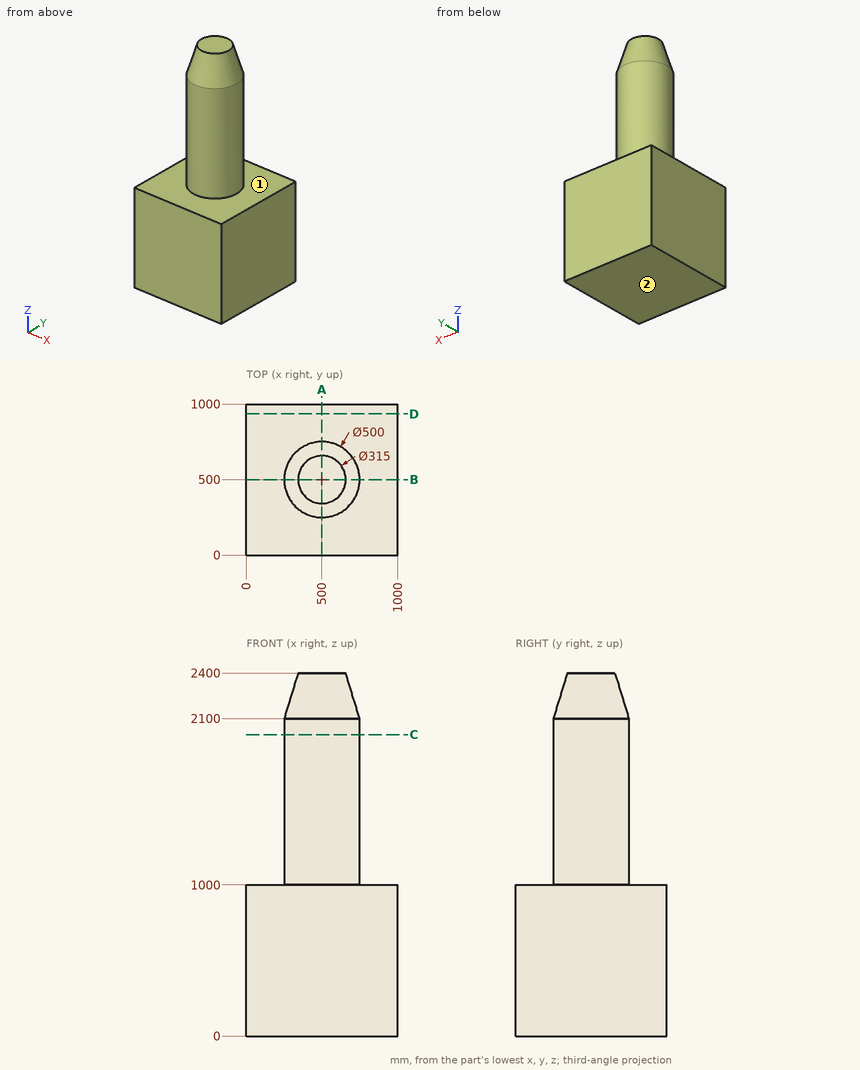
Check sheet for the drawn part. Datum: minimum x, y, z corner. Units: mm. A direction names the side the tool comes from. Give positions to 0.01 mm unless a question says otherwise; leave off trailing zeros. Order: outer loops, then holes, each group sorted by start corner. A loop starts at its lowest first (then second) coordinate and runs counter-clockwise, first axis right, second up. Notation, with made-up numbers: (78.5, 81) -> (131.5, 81) arc R20 ccw to (131.5, 86) -> close; hole circle Ø3 at (60, 47.5). An arc over 180 degrees is marked (long way). Return JSON: item names as keys, results as strings.
1. Cross-section at C-C, the plane z = 1993. Record the cut outline in (x, y), plus the area to 3 significant figures.
From the geometry:
{"outline": "circle Ø500 at (500, 500)", "area": "196,000 mm^2"}
2. Cross-section at A-A, the plane x = 500. Record the cut outline in (y, z).
From the geometry:
{"outline": "(0, 0) -> (1000, 0) -> (1000, 1000) -> (750, 1000) -> (750, 2100) -> (657.5, 2400) -> (342.5, 2400) -> (250, 2100) -> (250, 1000) -> (0, 1000) -> close"}
3. Material ranges on probe 1 along Z at (x, y) = (942, 428.5); probe 2 along X at (y, z) = (598.5, 1465); probe 3 along Y at (x, z) = (559, 1747.5), recorded low to high. Write a range as [from, to].
From the geometry:
{"probe 1": "[0, 1000]", "probe 2": "[270.22, 729.78]", "probe 3": "[257.06, 742.94]"}
4. Set-up check for the marked faces 1 and 2: record each of +Z, -Z, +X, -X, +Y, -Y from which the full face is reachable in a straight line by a thin tool's end or side.
From the geometry:
{"face 1": "+Z", "face 2": "-Z, +X, -X, +Y, -Y"}
5. Cross-section at D-D, the plane y = 935. Record the cut outline in (x, z), plus the area to 3 significant figures.
From the geometry:
{"outline": "(0, 0) -> (1000, 0) -> (1000, 1000) -> (0, 1000) -> close", "area": "1,000,000 mm^2"}
6. Go/stop test with flat-tipped pins: P1, Ø8, axis at x = 485, y = 590, coming from the -Z side; P2, Ø5, axis at x = 471.5, z = 1646, coming from the +Y side; P3, Ø5, axis at x = 723.5, y = 820, coming from the +Z side; P4, Ø8, axis at y = 323.5, z = 1905, coming from the +X side. Record where each tip stops, or that it passes through.
From the geometry:
{"P1": "z = 0", "P2": "y = 748.64", "P3": "z = 1000", "P4": "x = 680.95"}
